Model file for the job. Use its own axes, mm. Face numbers are marked on the shaded views. A direction names the side the tool comes from. Give positions to 0.01 mm unless a question says otherwise; leave off trailing zeros. Loops run counter-clockwise (first coordinate to the right, second up) from the corner with the lowest first, then second, coordinate; pieces in that order, holes last. Notation, with made-up numbers: M 54,-4.75 L 59,-4.75 A12 ccw 59,12.25 Z; hole C 59,42.5 d11. An arc over 180 degrees is marked long. Answer in a Markdown table with one row per item.
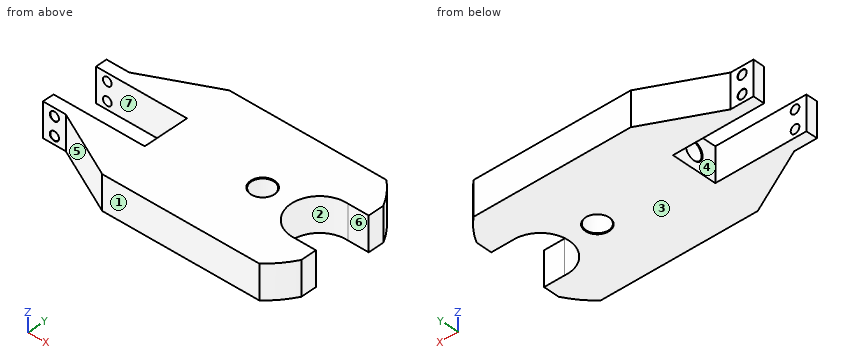
```python
from build123d import *

# Parameters (mm, degrees)
F1_DEPTH = 38.1


# Not quite as in the source:
# - a pattern or mirror of a feature is missing from the dataset's text; its kind, count and spacing are read off the source's solid


with BuildPart() as f1:
    # F0 (on Top) → F1 (new body)
    with BuildSketch(Plane.XY):
        with BuildLine():
            Line((0, 25.4), (0, 0))
            Line((0, 0), (0, -25.4))
            Line((0, -25.4), (-101.6, -25.4))
            Line((-101.6, -25.4), (-101.6, -38.1))
            Line((-101.6, -38.1), (-76.2, -38.1))
            Line((-76.2, -38.1), (-0.1165057322, -76.2))
            Line((-0.1165057322, -76.2), (175.152083301, -76.2))
            ThreePointArc((175.152083301, -76.2), (187.161060787, -63.6252139407), (196.85, -49.1868884968))
            Line((196.85, -49.1868884968), (196.85, -31.6608884968))
            Line((196.85, -31.6608884968), (173.8271074, -31.6608884968))
            ThreePointArc((173.8271074, -31.6608884968), (139.7, 0), (173.8271074, 31.6608884968))
            Line((173.8271074, 31.6608884968), (196.85, 31.6608884968))
            Line((196.85, 31.6608884968), (196.85, 49.1868884968))
            ThreePointArc((196.85, 49.1868884968), (187.161060787, 63.6252139407), (175.152083301, 76.2))
            Line((175.152083301, 76.2), (-0.1165057322, 76.2))
            Line((-0.1165057322, 76.2), (-76.2, 38.1))
            Line((-76.2, 38.1), (-101.6, 38.1))
            Line((-101.6, 38.1), (-101.6, 25.4))
            Line((-101.6, 25.4), (0, 25.4))
        make_face()
    extrude(amount=F1_DEPTH)

    # F3 (on offset) → F4 (revolve, cut)
    with BuildSketch(Plane(origin=(107.95, 0, 0), x_dir=(0, -1, 0), z_dir=(-1, 0, 0))):
        Polygon((-13.335, 0), (0, 0), (0, 38.1), (-13.335, 38.1), (-12.7, 37.465), (-12.7, 0.635), align=None)
    revolve(axis=Axis((107.95, 0, 19.05), (0, 0, 1)), mode=Mode.SUBTRACT)

    # F6 (on mid) → F7 (revolve, cut)
    with BuildSketch(Plane.XY.offset(19.05)):
        Polygon((24.7731973962, 0), (0, 0), (0, -10.16), (0.635, -9.525), (19.05, -9.525), align=None)
    revolve(axis=Axis((12.3865986981, 0, 19.05), (1, 0, 0)), mode=Mode.SUBTRACT)

    # F9 (on offset) → F10 (revolve, cut)
    with BuildSketch(Plane(origin=(-88.9, 0, 0), x_dir=(0, -1, 0), z_dir=(-1, 0, 0))):
        Polygon((38.1, 8.89), (-38.1, 8.89), (-38.1, 3.81), (-37.846, 4.064), (37.846, 4.064), (38.1, 3.81), align=None)
    f10 = revolve(axis=Axis((-88.9, 0, 8.89), (0, 1, 0)), mode=Mode.SUBTRACT)

    # F10_copies: F10 across plane
    add(f10.mirror(Plane.XY.offset(19.05)), mode=Mode.SUBTRACT)


solid = f1.part
```
Q1. Saw through at C-C (y = -21.5). Give the cut face in (x, z).
Reported:
| item | result |
|---|---|
| outline | M 0,0 L 148.09,0 L 148.09,38.1 L 0,38.1 Z |
Q2. Saw through at A-A (x = 107.95). Give the cut face in (y, z) (3 decimals).
Reported:
| item | result |
|---|---|
| outline | M -76.2,0 L -13.335,0 L -12.7,0.635 L -12.7,37.465 L -13.335,38.1 L -76.2,38.1 Z; M 12.7,0.635 L 13.335,0 L 76.2,0 L 76.2,38.1 L 13.335,38.1 L 12.7,37.465 Z |
Q3. 3-axis set-ups, long thin cutter, end or side, ignore diameter. For the marked faces 5, 6 and 7: which of +Z, -Z, +X, -X, +Y, -Y reach the whole face in a straight line?
Reported:
| item | result |
|---|---|
| face 5 | +Z, -Z, -X, -Y |
| face 6 | +Z, -Z, +X |
| face 7 | +Z, -Z, -X |
Q4. Mould opens along Y. For the marked faces 1, 2, 3 and 4 say: released by +Y, released by -Y, zero draft, split by the parting line, or undercut.
Reported:
| item | result |
|---|---|
| face 1 | released by -Y |
| face 2 | undercut |
| face 3 | zero draft |
| face 4 | undercut |
Q5. Drop flat-ended pins along their axis: pin 1 (11 mm diameter, centred on x = -88.9, z = 8.89, fed in from +Y); pin 2 (20.5 mm diameter, centred on x = -91, z = 22, fed in from -Y); pin 3 (7 mm diameter, centred on x = 189.5, z = 28, fed in from +Y). Give the stop position or say it passes through.
Reported:
| item | result |
|---|---|
| pin 1 | y = 38.1 |
| pin 2 | y = -38.1 |
| pin 3 | y = 65.04 |
Q6. Saw through at B-B (x = -26). Give the cut face in (y, z), and give its area (3 significant figures).
Reported:
| item | result |
|---|---|
| outline | M -63.24,0 L -25.4,0 L -25.4,38.1 L -63.24,38.1 Z; M 25.4,0 L 63.24,0 L 63.24,38.1 L 25.4,38.1 Z |
| area | 2,880 mm² |
Q7. Probe probe 1 along Z at (x, y) = (-88.9, 29.25); probe 2 along X at (y, z) = (-35, 29.21); probe 3 along Z at (x, y) = (12.25, 0) (3 decimals). List the from-to ranges inside material, lowest first.
Reported:
| item | result |
|---|---|
| probe 1 | 0 to 4.06, 13.72 to 24.38, 34.04 to 38.1 |
| probe 2 | -101.6 to -93.73, -84.07 to 196.85 |
| probe 3 | 0 to 9.525, 28.575 to 38.1 |
